Design review of the part built by this model. Coordinates are the model's own, in mm. A direction names the side the tool comes from. Give positions to 0.01 mm unless a question says otherwise; leave off trailing zeros. Write each loop counter-clockwise with the first axis right and the second up, starting at its lowest first coordinate (ties: lowest second). Pieces come first, ordered by that corner, then holes.
```python
from build123d import *

# Parameters (mm, degrees)
SKETCH_2_R           = 5
EXTRUDE_3_DEPTH      = 5
EXTRUDE_4_DEPTH      = 3
EXTRUDE_4_DEPTH_BACK = 3
SKETCH_4_W           = 5
SKETCH_4_H           = 6
EXTRUDE_5_DEPTH      = 3
SKETCH_5_W           = 5
SKETCH_5_H           = 6
EXTRUDE_6_DEPTH      = 3
SKETCH_6_R           = 2.5
CUT_EXTRUDE_1_DEPTH  = 5
EXTRUDE_START        = -5
SKETCH_7_R           = 2.25
EXTRUDE_7_DEPTH      = 8


with BuildPart() as part:
    # Sketch 2 → Extrude 3 (new body)
    with BuildSketch(Plane.XY):
        Circle(SKETCH_2_R)
    extrude(amount=EXTRUDE_3_DEPTH)



with BuildPart() as body_2:
    # Sketch 3 → Extrude 4 (new, two sides: drawn at the far end of the back side and taken through both)
    with BuildSketch(Plane(origin=(0, 0, 0), x_dir=(1, 0, 0), z_dir=(0, 1, 0)).offset(-EXTRUDE_4_DEPTH_BACK)):
        with BuildLine():
            ThreePointArc((5, 0), (22.079402166, -12.252451216), (24.150635095, -33.169872981))
            Line((24.150635095, -33.169872981), (19.820508076, -30.669872981))
            ThreePointArc((19.820508076, -30.669872981), (17.853571071, -14.692235936), (5, -5))
            Line((5, -5), (5, 0))
        make_face()
    extrude(amount=EXTRUDE_4_DEPTH + EXTRUDE_4_DEPTH_BACK)



with BuildPart() as body_3:
    # Sketch 3_3 → Revolve 1 (revolve)
    with BuildSketch(Plane(origin=(0, 0, 0), x_dir=(1, 0, 0), z_dir=(0, 1, 0)), mode=Mode.PRIVATE) as revolve_1_sk:
        Polygon((24.150635095, -33.169872981), (19.820508076, -30.669872981), (17.320508076, -35), (21.650635095, -37.5), align=None)
    revolve(revolve_1_sk.sketch.rotate(Axis((0, 0, 25), (0.8660254037844406, 0, 0.4999999999999967)), 180), axis=Axis((0, 0, 25), (0.8660254037844406, 0, 0.4999999999999967)))


with BuildPart() as body_2_1:
    add(body_2.part)

    add(body_3.part)  # Extrude 5 merges body 3
    # Sketch 4 → Extrude 5 (add)
    with BuildSketch(Plane(origin=(-8.325317547, 0, 14.419872981), x_dir=(0.8660254037844396, 0, 0.49999999999999856), z_dir=(-0.49999999999999856, 0, 0.8660254037844396))):
        with Locations((35, 0)):
            Rectangle(SKETCH_4_W, SKETCH_4_H)
    extrude(amount=EXTRUDE_5_DEPTH)


with BuildPart() as part_1:
    add(part.part)

    add(body_2_1.part)  # Extrude 6 merges body 2
    # Sketch 5 → Extrude 6 (add)
    with BuildSketch(Plane.ZY.offset(-5)):
        with Locations((2.5, 0)):
            Rectangle(SKETCH_5_W, SKETCH_5_H)
    extrude(amount=EXTRUDE_6_DEPTH)

    # Sketch 6 → Cut-Extrude 1 (cut)
    with BuildSketch(Plane(origin=(28.145825623, 0, 16.25), x_dir=(-0.49999999999999856, 0, 0.8660254037844396), z_dir=(-0.8660254037844396, 0, -0.49999999999999856))):
        with Locations((21.650635095, 0)):
            Circle(SKETCH_6_R)
    extrude(amount=-CUT_EXTRUDE_1_DEPTH, mode=Mode.SUBTRACT)

    # Sketch 7 → Extrude 7 (add)
    with BuildSketch(Plane.XY.offset(5).offset(EXTRUDE_START)):
        Circle(SKETCH_7_R)
    extrude(amount=-EXTRUDE_7_DEPTH)


solid = part_1.part
```
(1) Clearance check with flat-ended pins moving along their axes: P1, Ø3, axis at x = 0, y = -1.5, coming from the +Z side; P2, Ø6.5, axis at x = 16.5, z = 12.5, coming from the -Y side; P3, Ø1, axis at x = 3, y = -2, coming from the -Z side. State where each tip first meets the part, or that it passes through.
Resolved:
P1: stops at z = 5
P2: stops at y = -3
P3: stops at z = 0
(2) Consider section D-D, the plane z = 15. Give the boundary of the cut face in (x, y).
Resolved:
outline: (18.03, -3) - (23.45, -3) - (23.45, 3) - (18.03, 3) - close
(3) Consider section B-B, the plane x = 0. Give the boundary of the cut face in (y, z).
Resolved:
outline: (-5, 0) - (-2.25, 0) - (-2.25, -8) - (2.25, -8) - (2.25, 0) - (5, 0) - (5, 5) - (-5, 5) - close
(4) Consider section C-C, the plane y = -3.5. Give the boundary of the cut face in (x, z).
Resolved:
outline: (-3.57, 0) - (3.57, 0) - (3.57, 5) - (-3.57, 5) - close; (15.54, 38.09) - (19.11, 31.91) - (23.44, 34.41) - (19.87, 40.59) - close
(5) Consider section A-A, the plane y = 0.75. Give the boundary of the cut face in (x, z), then the cut area to 3 significant figures.
Resolved:
outline: (-4.94, 0) - (-2.12, 0) - (-2.12, -8) - (2.12, -8) - (2.12, 0) - (5, 0) arc R25.5 ccw to (24.15, 33.17) - (22.84, 35.43) - (18.51, 32.93) - (19.82, 30.67) arc R20.62 cw to (5, 5) - (-4.94, 5) - close; (14.85, 39.28) - (16.13, 37.07) - (20.46, 39.57) - (19.18, 41.78) - close
area: 296 mm2
(6) To check wall thickness, follow L1, parallel to X at y = -0.25, z = 24.5; L2, parallel to Z at x = 2, y = 1.75; L3, parallel to Z at x = 1, y = -0.25. State the ranges of each line that lie inside material, in increasing order.
Resolved:
L1: x = 20.61 to 25.49
L2: z = 0 to 5
L3: z = -8 to 5
(7) Tool access review of faces 4 (the face through (18, 3, 14)), 5 (the face through (-0.29, 2.23, -3.94)), 6 (the face through (0, 0, 5)): name each direction out of +Z, -Z, +X, -X, +Y, -Y from which nothing blocks a thin tool from reaching the whole face with its end or side.
Resolved:
face 4: -Z, +X, +Y
face 5: -Z
face 6: +Z, -X, +Y, -Y
(8) Mouldability with a two-part tool opening along Z and no side actions: class faces 1 (the face through (22.727, 2.152, 35.636)), 2 (the face through (-5, 0, 2)), 3 (the face through (17.968, -0.042, 14.893)) as pulls with the +Z half, pulls with the -Z half, needs draft (parallel to the pull), parting line crosses it, or undercut.
Resolved:
face 1: pulls with the +Z half
face 2: needs draft
face 3: undercut
